CAD build for the part. Positions are in the model's coordinates, mm. Face numbers are marked on the shaded views. A direction names the side the tool comes from. Give positions to 0.01 mm unless a question says otherwise; leave off trailing zeros. Write each loop counter-clockwise with the first axis right and the second up, starting at its lowest first coordinate (ties: lowest second). Pieces come first, ordered by that corner, then holes. Notation, with made-up numbers: M 27.5,72 L 86.5,72 A26 cw 86.5,106 Z; hole C 76,35 d1. An arc over 180 degrees is marked long. One line per question, with ' | ' between items. Start each with the question number.
1. Which spindle directions (+Z, -Z, +X, -X, +Y, -Y) get a long thin tool onto all of the face, cutting with end or side? Do the marked faces 4, 5 and 6. Say none if no direction does.
2. Cut at A-A, the plane y = 2.75. Write the cut outline in (x, z).
3. Flat gauge pins, fed straight in: pin 1 (0.5 mm diameter, centred on x = 12, y = 7.5, fed in from -Z); pin 2 (2 mm diameter, centred on y = 9, z = 4, fed in from -X); pin 3 (1.6 mm diameter, centred on y = 1, z = -3, fed in from +X). Where does each tip first touch, or does it go through?
4. Cut at B-B, the plane z = 1.5. Write the cut outline in (x, y).
5. Wall check: L1, parallel to X at y = 6.75, z = 1; L2, parallel to Y at x = 9, z = -2; L3, parallel to Y at x = 12.75, z = 0.25. Give the ranges that are in metal, low to high.
6. Pull direction Z, two halves, no side cores. Call the marked faces 1, 2 and 3: released by +Z, released by -Z, zero draft, split by the parting line, or undercut.
7. Cut at D-D, the plane y = 9.5. Write the cut outline in (x, z).
8. Cut at C-C, the plane x = 1.25. Write the cut outline in (y, z), then the cut area to 3 significant figures.
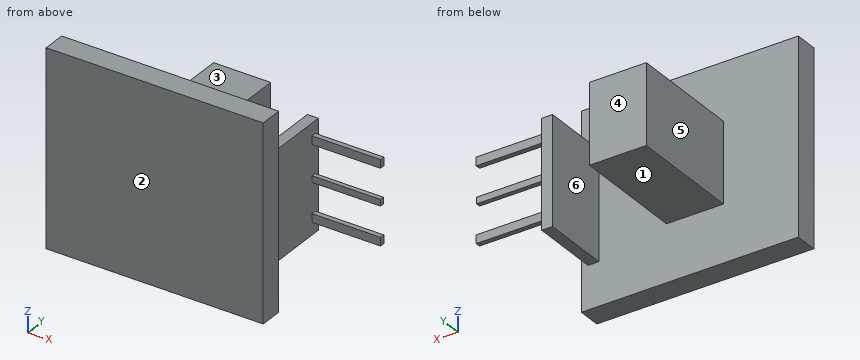
```python
from build123d import *

# Parameters (mm, degrees)
ESQUISSE1_W        = 19
ESQUISSE1_H        = 17
BOSS_EXTRU_1_DEPTH = 2
ESQUISSE2_W        = 0.955718941
ESQUISSE2_H        = 9.466168562
BOSS_EXTRU_2_DEPTH = 6
ESQUISSE3_W        = 0.738510091
ESQUISSE3_H        = 0.422005766
BOSS_EXTRU_3_DEPTH = 6
ESQUISSE4_W        = 0.562674356
ESQUISSE4_H        = 0.386838619
BOSS_EXTRU_4_DEPTH = 6
ESQUISSE5_W        = 5
ESQUISSE5_H        = 7
BOSS_EXTRU_5_DEPTH = 10


with BuildPart() as part:
    # Esquisse1 → Boss.-Extru.1 (new body)
    with BuildSketch(Plane(origin=(0, 0, 0), x_dir=(1, 0, 0), z_dir=(0, 1, 0))):
        Rectangle(ESQUISSE1_W, ESQUISSE1_H)
    extrude(amount=BOSS_EXTRU_1_DEPTH)

    # Esquisse2 → Boss.-Extru.2 (add)
    with BuildSketch(Plane(origin=(0, 2, 0), x_dir=(1, 0, 0), z_dir=(0, 1, 0))):
        with Locations((8.442183982, 0)):
            Rectangle(ESQUISSE2_W, ESQUISSE2_H)
    extrude(amount=BOSS_EXTRU_2_DEPTH)

    # Esquisse3 → Boss.-Extru.3 (add)
    with BuildSketch(Plane(origin=(8.920043452, 0, 0), x_dir=(0, 0, -1), z_dir=(1, 0, 0))):
        with Locations((-3.288128263, 7.393629704)):
            Rectangle(ESQUISSE3_W, ESQUISSE3_H)
    boss_extru_3 = extrude(amount=BOSS_EXTRU_3_DEPTH)

    # Symétrie1: Boss.-Extru.3 across plane
    add(boss_extru_3.mirror(Plane.XY))

    # Esquisse4 → Boss.-Extru.4 (add)
    with BuildSketch(Plane(origin=(8.920043452, 0, 0), x_dir=(0, 0, -1), z_dir=(1, 0, 0))):
        with Locations((0, 7.376046131)):
            Rectangle(ESQUISSE4_W, ESQUISSE4_H)
    extrude(amount=BOSS_EXTRU_4_DEPTH)

    # Esquisse5 → Boss.-Extru.5 (add)
    with BuildSketch(Plane(origin=(0, 2, 0), x_dir=(1, 0, 0), z_dir=(0, 1, 0))):
        with Locations((-0.447844474, 0.014350287)):
            Rectangle(ESQUISSE5_W, ESQUISSE5_H)
    extrude(amount=BOSS_EXTRU_5_DEPTH)


solid = part.part
```
Here are the results:
1) face 4: +Z, -Z, +X, -X, +Y | face 5: +Z, -Z, -X, +Y | face 6: +Z, -Z, +Y
2) outline: M -2.95,-3.51 L 2.05,-3.51 L 2.05,3.49 L -2.95,3.49 Z; M 7.96,-4.73 L 8.92,-4.73 L 8.92,4.73 L 7.96,4.73 Z
3) pin 1: z = -3.66 | pin 2: x = -2.95 | pin 3: x = 9.5
4) outline: M -9.5,0 L 9.5,0 L 9.5,2 L 8.92,2 L 8.92,8 L 7.96,8 L 7.96,2 L 2.05,2 L 2.05,12 L -2.95,12 L -2.95,2 L -9.5,2 Z
5) L1: -2.95 to 2.05, 7.96 to 8.92 | L2: 0 to 2 | L3: 7.18 to 7.57
6) face 1: released by -Z | face 2: zero draft | face 3: released by +Z
7) outline: M -2.95,-3.51 L 2.05,-3.51 L 2.05,3.49 L -2.95,3.49 Z
8) outline: M 0,-8.5 L 2,-8.5 L 2,-3.51 L 12,-3.51 L 12,3.49 L 2,3.49 L 2,8.5 L 0,8.5 Z | area: 104 mm^2
